Design review of the part shown in the three views and the two pictorial views. Dimensions are in mm from the part's minimum x, y and z. A direction names the side the tool comes from. Round coordinates to 2 decimals unless told otherwise and drop trailing zeros. Loops run counter-clockwise (first coordinate to the right, second up) from the corner with the lowest first, then second, coordinate; pieces in that order, holes last. Notation, with made-up numbers: M 21,3 L 68,3 A16 ccw 68,15 Z; hole C -8,34 d7. An arc over 180 degrees is marked long. Answer as CSV lines item,"result". Start each with the question number.
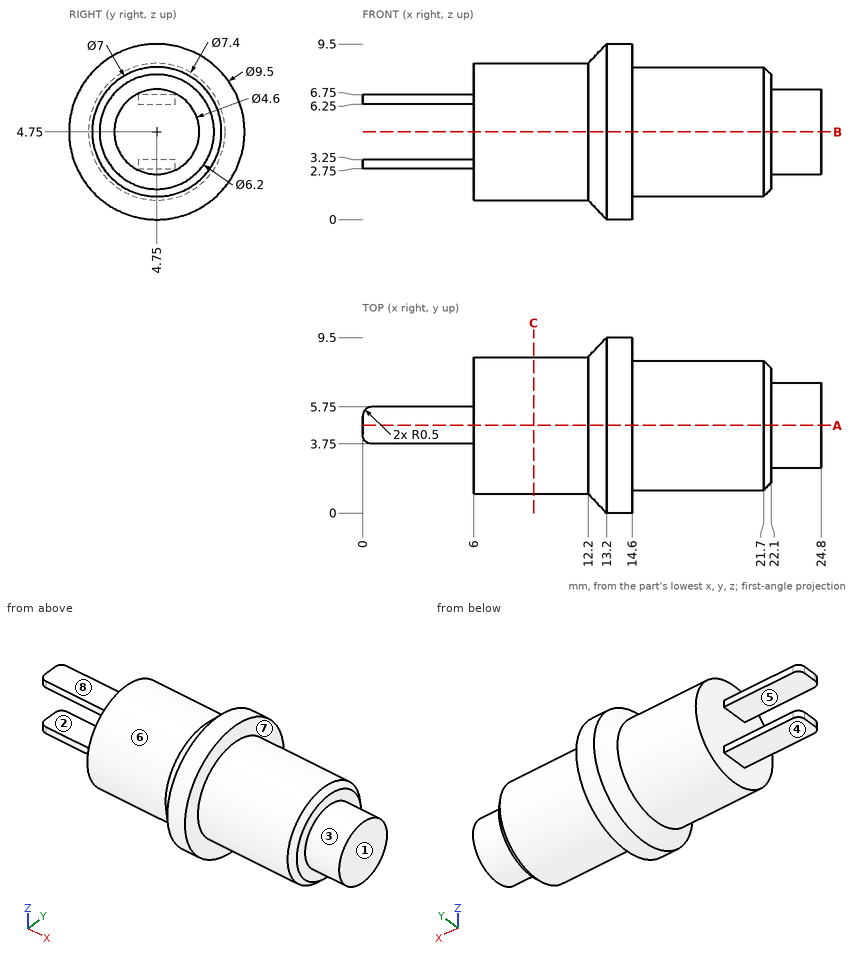
Item 1: Consider section B-B, the plane z = 4.75. Write out the cut boundary in (x, y).
Item 2: Consider section C-C, the plane x = 9.25. Write out the cut boundary in (y, z), then the cut area to 3 significant figures.
Item 3: To check wall thickness, follow line 1 (Z direction, x = 1.5, y = 4.25); line 2 (X direction, y = 2.75, z = 6.25); line 3 (Z direction, x = 9.75, y = 1.5). State the ranges of each line that lie inside material, in increasing order.
Item 4: The part is to be moulded in two halves that separate along Z. For the marked faces 5, 6, 7 and 8, say which applies: +Z half, -Z half, draft (parallel to the pull), parting line (faces both ways), or undercut.
Item 5: Tool access review of the marked faces 1, 2, 3 and 4: name each direction out of +Z, -Z, +X, -X, +Y, -Y from which nothing blocks a thin tool from reaching the whole face with its end or side.
Item 6: Consider section A-A, the plane y = 4.75. Write out the cut boundary in (x, z), then the cut area to 3 significant figures.
Item 7: Insertion check: pin 1 Ø1 at (x, y) = (3, 4.5) entering from +Z; pin 2 Ø0.6 at (x, z) = (3, 6.5) entering from -Y; pin 3 Ø5 at (x, z) = (20.5, 5) entering from +Y. Each pin has a flat end and moves straight along its axis. Give the tip position at first contact, or say it passes through.
Found:
1,outline,"M 6,1.05 L 12.2,1.05 L 13.2,0 L 14.6,0 L 14.6,1.25 L 21.7,1.25 L 22.1,1.65 L 22.1,2.45 L 24.8,2.45 L 24.8,7.05 L 22.1,7.05 L 22.1,7.85 L 21.7,8.25 L 14.6,8.25 L 14.6,9.5 L 13.2,9.5 L 12.2,8.45 L 6,8.45 Z"
2,outline,"C 4.75,4.75 d7.4"
2,area,"43.0 mm^2"
3,line 1,"z = 2.75 to 3.25, 6.25 to 6.75"
3,line 2,"x = 6 to 22.1"
3,line 3,"z = 2.98 to 6.52"
4,face 5,"undercut"
4,face 6,"parting line"
4,face 7,"draft"
4,face 8,"+Z half"
5,face 1,"+Z, -Z, +X, +Y, -Y"
5,face 2,"-X, +Y, -Y"
5,face 3,"+X"
5,face 4,"-Z, -X, +Y, -Y"
6,outline,"M 0,2.75 L 6,2.75 L 6,1.05 L 12.2,1.05 L 13.2,0 L 14.6,0 L 14.6,1.25 L 21.7,1.25 L 22.1,1.65 L 22.1,2.45 L 24.8,2.45 L 24.8,7.05 L 22.1,7.05 L 22.1,7.85 L 21.7,8.25 L 14.6,8.25 L 14.6,9.5 L 13.2,9.5 L 12.2,8.45 L 6,8.45 L 6,6.75 L 0,6.75 L 0,6.25 L 6,6.25 L 6,3.25 L 0,3.25 Z"
6,area,"138 mm^2"
7,pin 1,"stops at z = 6.75"
7,pin 2,"stops at y = 3.75"
7,pin 3,"stops at y = 8.25"
